from build123d import *

# Parameters (mm, degrees)
SKETCH_1_R          = 1
SKETCH_1_R_2        = 1.5
EXTRUDE_1_DEPTH     = 3
SKETCH_2_W          = 8
SKETCH_2_H          = 0.5
CUT_EXTRUDE_1_DEPTH = 10
FILLET_1_R          = 2


with BuildPart() as part:
    # 草图1 → 凸台-拉伸1 (new body)
    with BuildSketch(Plane(origin=(0, 0, 0), x_dir=(1, 0, 0), z_dir=(0, 1, 0))):
        Polygon((-17.5, 2.5), (-17.5, -9), (17.5, -9), (17.5, 9), (-1.5, 9), (-1.5, 2.5), align=None)
        with Locations(Location((-14, -6, 0), (0, 0, 270))):
            Circle(SKETCH_1_R, mode=Mode.SUBTRACT)
        with Locations(Location((2.5, -4, 0), (0, 0, 270))):
            Circle(SKETCH_1_R_2, mode=Mode.SUBTRACT)
        with Locations(Location((-14, 0, 0), (0, 0, 270))):
            Circle(SKETCH_1_R, mode=Mode.SUBTRACT)
        with Locations(Location((2.5, 4, 0), (0, 0, 270))):
            Circle(SKETCH_1_R_2, mode=Mode.SUBTRACT)
    extrude(amount=EXTRUDE_1_DEPTH)

    # 草图2 → 切除-拉伸1 (cut)
    with BuildSketch(Plane(origin=(0, 3, 0), x_dir=(1, 0, 0), z_dir=(0, 1, 0))):
        with Locations((2.5, 8.75)):
            Rectangle(SKETCH_2_W, SKETCH_2_H)
        Polygon((17.5, -9), (17.5, 9), (6.5, 9), (6.5, 8.5), (6.5, -9), align=None)
    extrude(amount=-CUT_EXTRUDE_1_DEPTH, mode=Mode.SUBTRACT)

    # 圆角1
    fillet_1_edges = [part.edges().sort_by_distance(p)[0] for p in [
        (-17.5, 1.5, 9),
        (-17.5, 1.5, -2.5),
        (-1.5, 1.5, -2.5),
        (-1.5, 1.5, -8.5),
        (6.5, 1.5, 9),
        (6.5, 1.5, -8.5),
    ]]
    fillet(fillet_1_edges, radius=FILLET_1_R)


solid = part.part
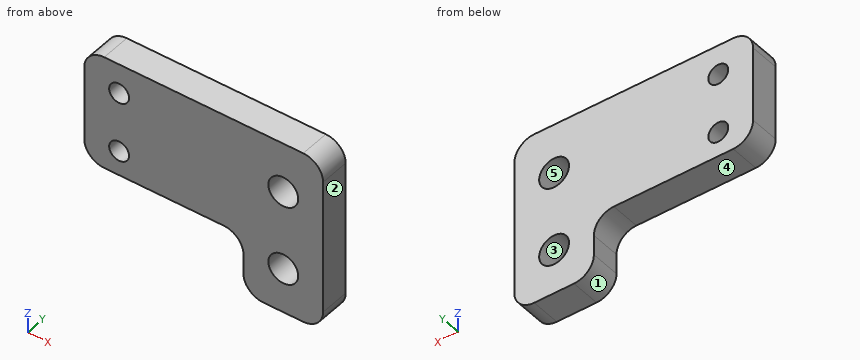
Verification items for the finished model (mm, model axes). Face numbers are marked on the shaded views. A direction names the side the tool comes from. Give positions to 0.01 mm unless a question says otherwise; leave off trailing zeros. Order: outer loops, then holes, each group sorted by start corner. A loop starts at its lowest first (then second) coordinate and runs counter-clockwise, first axis right, second up. Notation, with made-up numbers: (-16.75, -22) -> (42.25, -22) arc R21 cw to (42.25, -10) -> close; hole circle Ø2 at (37.25, 4). An arc over 180 degrees is marked (long way). Answer as CSV lines item,"result".
Q1. Access from +Z, -Z, +X, -X, +Y, -Y to the whole of each face (thin tool, end or side, straight path). Record for the marked faces 4 and 5.
Solutions:
face 4,"-Z, -X, +Y, -Y"
face 5,"+Y, -Y"
Q2. Sectioned sample at C-C on y = 1.05. Record the cut outline in (x, z), plus the area to 3 significant figures.
Solutions:
outline,"(-17.5, -0.5) arc R2 ccw to (-15.5, -2.5) -> (-3.5, -2.5) arc R2 cw to (-1.5, -4.5) -> (-1.5, -6.5) arc R2 ccw to (0.5, -8.5) -> (4.5, -8.5) arc R2 ccw to (6.5, -6.5) -> (6.5, 7) arc R2 ccw to (4.5, 9) -> (-15.5, 9) arc R2 ccw to (-17.5, 7) -> close; hole circle Ø2 at (-14, 0); hole circle Ø2 at (-14, 6); hole circle Ø3 at (2.5, -4); hole circle Ø3 at (2.5, 4)"
area,"300 mm²"
Q3. Scan lines: probe 1 along X at (y, z) = (1.7, 6); probe 2 along Z at (x, y) = (-14.5, 1.5); probe 3 along X at (y, z) = (0.9, 4). Record each from-to range of solid material in increasing order.
Solutions:
probe 1,"x = -17.5 to -15, -13 to 6.5"
probe 2,"z = -2.5 to -0.87, 0.87 to 5.13, 6.87 to 9"
probe 3,"x = -17.5 to 1, 4 to 6.5"
Q4. Sectioned sample at B-B on x = 2.5. Record the cut outline in (y, z), plus the area to 3 significant figures.
Solutions:
outline,"(0, -8.5) -> (3, -8.5) -> (3, -5.5) -> (0, -5.5) -> close; (0, -2.5) -> (3, -2.5) -> (3, 2.5) -> (0, 2.5) -> close; (0, 5.5) -> (3, 5.5) -> (3, 9) -> (0, 9) -> close"
area,"34.5 mm²"
Q5. Release check for a two-part mould opening along X. For the marked faces 1, 2 and 3 record: +X half, -X half, draft (parallel to the pull), parting line (faces both ways), or undercut.
Solutions:
face 1,"-X half"
face 2,"+X half"
face 3,"undercut"
Q6. Sectioned sample at A-A on z = 0. Record the cut outline in (x, y).
Solutions:
outline,"(-17.5, 0) -> (-15, 0) -> (-15, 3) -> (-17.5, 3) -> close; (-13, 0) -> (6.5, 0) -> (6.5, 3) -> (-13, 3) -> close"
Q7. Sectioned sample at D-D on x = -14. Record the cut outline in (y, z), plus the area to 3 significant figures.
Solutions:
outline,"(0, -2.5) -> (3, -2.5) -> (3, -1) -> (0, -1) -> close; (0, 1) -> (3, 1) -> (3, 5) -> (0, 5) -> close; (0, 7) -> (3, 7) -> (3, 9) -> (0, 9) -> close"
area,"22.5 mm²"
Q8. Depth check by flat-ended pin: pin 1 (1.6 mm diameter, centred on y = 1.5, z = -5, fed in from -X); pin 2 (0.9 mm diameter, centred on x = -10, y = 1, fed in from -Z). Enter the tip coordinate at first touch or a pass-through.
Solutions:
pin 1,"stops at x = -1.52"
pin 2,"stops at z = -2.5"
